The model under review builds one solid part; all positions refer to its coordinate system, in mm. Face numbers are marked on the shaded views. A direction names the side the tool comes from. Give positions to 0.01 mm unless a question says otherwise; leave off trailing zeros. Order: outer loops, then holes, each group sorted by start corner. A loop starts at its lowest first (then second) coordinate and runs counter-clockwise, first axis right, second up. Notation, with made-up numbers: (19, 54) - (63, 54) arc R9 ccw to (63, 60) - close; hole circle Ø8 at (15.25, 85). An arc over 180 degrees is marked (long way). Use CSV: the item, a comma, the result in double quotes. Start each with the question number.
1. Take a section at A-A, the plane y = 1.5. Count the separate pieces of the cut face and the enclosed holes in it, then the cut area to 3 significant figures.
2. For pin 1 (2 mm diameter, centred on y = -8, z = 72, fed in from -X); pin 2 (5 mm diameter, centred on y = 2, z = 59, fed in from -X); pin 3 (10 mm diameter, centred on x = -27, y = -5, fed in from +Z); pin 4 (17.5 mm diameter, centred on x = -56, z = 6.5, fed in from +Y), all flat-tipped, find the tip position at first contact; note any pin that passes through.
3. Machinability: for the marked faces 1 and 2, which of the approach directions +Z, -Z, +X, -X, +Y, -Y give a long, thin tool a straight path to every point of the face, cutting with its end or side? Answer none if there is none.
4. Take a section at B-B, the plane z = 36. State the section outline as (x, y) points (1 decimal), then the cut area to 3 significant figures.
5. To check wall thickness, follow line 1 (Y direction, x = -54, z = -56) (3 decimals); line 2 (Y direction, x = -55.5, z = -52) (3 decimals); line 3 (Z direction, x = -9.5, y = 5.5) (3 decimals). State the ranges of each line that lie inside material, in increasing order. Write a range as [from, to].
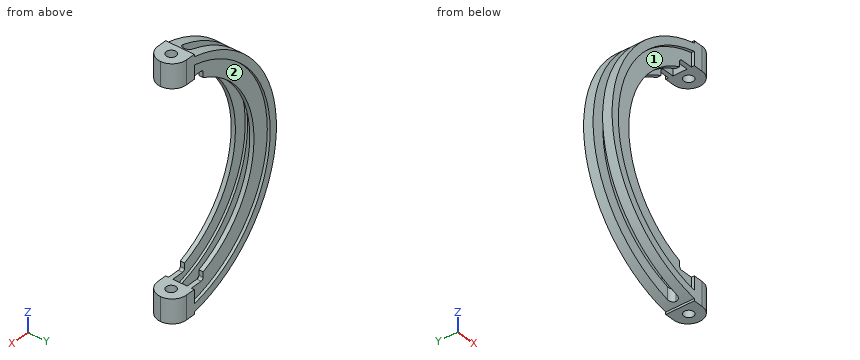
```python
from build123d import *

# Parameters (mm, degrees)
F3_W        = 19.05
F3_H        = 15.875
F4_DEPTH    = 15.875
F6_D        = 6.5278
F8_DEPTH    = 165.101
F9_T1_DEPTH = 63.5
F9_T3_DEPTH = 63.5
F11_DEPTH   = 17.1460001


# Not quite as in the source:
# - a fillet or chamfer that OpenCascade refuses, or shapes differently, is made with other operations: its cross-section is extruded or revolved along the edge and cut away or added


with BuildPart() as f2:
    # F2: sweep along a path in F0
    with BuildLine(Plane.XZ) as f2_path:
        ThreePointArc((0, 76.2), (-76.2, 0), (0, -76.2))
    # F1 (on Right) → F2 (sweep)
    with BuildSketch(Plane.YZ):
        Polygon((9.525, 82.55), (0, 82.55), (-9.525, 82.55), (-9.525, 77.47), (-7.62, 77.47), (-7.62, 66.675), (-4.7625, 66.675), (-4.7625, 74.6125), (0, 74.6125), (4.7625, 74.6125), (4.7625, 66.675), (7.62, 66.675), (7.62, 77.47), (9.525, 77.47), align=None)
    sweep(path=f2_path.line)

    # F3 (on face) → F4 (join)
    with BuildSketch(Plane.YZ):
        with Locations((0, 74.6125)):
            Rectangle(F3_W, F3_H)
        with Locations((0, -74.6125)):
            Rectangle(F3_W, F3_H)
    extrude(amount=-F4_DEPTH)

    # F6 (through all)
    with Locations(Plane.XY.offset(82.55)):
        with Locations((-8.73125, 0)):
            Hole(F6_D / 2)

    # F7 (on face) → F8 (cut, through all)
    with BuildSketch(Plane.XY.offset(82.55)):
        with BuildLine():
            Line((-22.225, 3.175), (-114.3, 3.175))
            Line((-114.3, 3.175), (-114.3, -3.175))
            Line((-114.3, -3.175), (-22.225, -3.175))
            ThreePointArc((-22.225, -3.175), (-19.9799359697, -2.2450640303), (-19.05, 0))
            ThreePointArc((-19.05, 0), (-19.9799359697, 2.2450640303), (-22.225, 3.175))
        make_face()
    extrude(amount=-F8_DEPTH, mode=Mode.SUBTRACT)

    # F9: fillet of radius 9.525 on 4 edges, made by hand

    # F9_s2 → F9_t1 (cut)
    with BuildSketch(Plane.XY.offset(42.8625)):
        with BuildLine():
            ThreePointArc((0, 0), (-2.7898079092, -6.7351920908), (-9.525, -9.525))
            Line((-9.525, -9.525), (0, -9.525))
            Line((0, -9.525), (0, 0))
        make_face()
        with BuildLine():
            ThreePointArc((0, 0), (-2.7898079092, 6.7351920908), (-9.525, 9.525))
            Line((-9.525, 9.525), (0, 9.525))
            Line((0, 9.525), (0, 0))
        make_face()
    extrude(amount=F9_T1_DEPTH, mode=Mode.SUBTRACT)

    # F9_s4 → F9_t3 (cut)
    with BuildSketch(Plane.XY.offset(-106.3625)):
        with BuildLine():
            ThreePointArc((-9.525, -9.525), (-2.7898079092, -6.7351920908), (0, 0))
            Line((0, 0), (0, -9.525))
            Line((0, -9.525), (-9.525, -9.525))
        make_face()
        with BuildLine():
            ThreePointArc((-9.525, 9.525), (-2.7898079092, 6.7351920908), (0, 0))
            Line((0, 0), (0, 9.525))
            Line((0, 9.525), (-9.525, 9.525))
        make_face()
    extrude(amount=F9_T3_DEPTH, mode=Mode.SUBTRACT)

    # F10 (on face) → F11 (cut, through all)
    with BuildSketch(Plane.XZ.offset(7.62)):
        with BuildLine():
            Line((0, 60.325), (0, 66.675))
            Line((0, 66.675), (-23.8125, 66.675))
            ThreePointArc((-23.8125, 66.675), (-24.9350320151, 66.2100320151), (-25.4, 65.0875))
            Line((-25.4, 65.0875), (-25.4, 60.325))
            Line((-25.4, 60.325), (0, 60.325))
        make_face()
        with BuildLine():
            Line((-23.8125, -66.675), (0, -66.675))
            Line((0, -66.675), (0, -60.325))
            Line((0, -60.325), (-25.4, -60.325))
            Line((-25.4, -60.325), (-25.4, -65.0875))
            ThreePointArc((-25.4, -65.0875), (-24.9350320151, -66.2100320151), (-23.8125, -66.675))
        make_face()
    extrude(amount=-F11_DEPTH, mode=Mode.SUBTRACT)


solid = f2.part
```
Determined:
1,separate pieces,"4"
1,enclosed holes,"0"
1,area,"374 mm²"
2,pin 1,"stops at x = -42.11"
2,pin 2,"stops at x = -59.91"
2,pin 3,"stops at z = 79.56"
2,pin 4,"passes through"
3,face 1,"-Y"
3,face 2,"+Y"
4,outline,"(-74.3, -9.5) - (-68.6, -9.5) - (-68.6, -7.6) - (-56.1, -7.6) - (-56.1, -4.8) - (-65.4, -4.8) - (-65.4, -3.2) - (-74.3, -3.2) - close; (-74.3, 3.2) - (-65.4, 3.2) - (-65.4, 4.8) - (-56.1, 4.8) - (-56.1, 7.6) - (-68.6, 7.6) - (-68.6, 9.5) - (-74.3, 9.5) - close"
4,area,"154 mm²"
5,line 1,"y = [-9.525, -3.175], [3.175, 9.525]"
5,line 2,"y = [-7.62, -3.175], [3.175, 7.62]"
5,line 3,"z = [-82.55, -66.675], [66.675, 82.55]"
